```python
from build123d import *

# Parameters (mm, degrees)
BOSS_EXTRU_1_DEPTH           = 38
BOSS_EXTRU_1_DEPTH_BACK      = 10
ESQUISSE8_W                  = 200
ESQUISSE8_H                  = 45
ENL_V_MAT_EXTRU_4_DEPTH      = 34
TROU_TARAUD_M14X1_51_D       = 12.5
TROU_TARAUD_M14X1_51_DEPTH   = 17.5
TROU_TARAUD_M14X1_51_TIP     = 3.755378869
ESQUISSE10_W                 = 99
ESQUISSE10_H                 = 34
ENL_V_MAT_EXTRU_6_DEPTH      = 14
CONG_2_R                     = 10
ENL_V_MAT_EXTRU_7_DEPTH      = 1
ENL_V_MAT_EXTRU_7_DEPTH_BACK = 49
TROU_TARAUD_M12X1_251_D      = 10.8
CHANFREIN1_SIZE              = 3
CONG_3_R                     = 1
ESQUISSE14_W                 = 218.12810102
ESQUISSE14_H                 = 78.447864133
ENL_V_MAT_EXTRU_8_DEPTH      = 1


with BuildPart() as part:
    # Esquisse1 → Boss.-Extru.1 (new body, two sides)
    with BuildSketch(Plane(origin=(0, 0, 0), x_dir=(1, 0, 0), z_dir=(0, 1, 0))) as boss_extru_1_sk:
        with BuildLine():
            Line((-7.5, 31), (149.5, 31))
            Line((149.5, 31), (149.5, 17.146428199))
            ThreePointArc((149.5, 17.146428199), (150.241799002, 13.366783469), (152.357142857, 10.147886077))
            ThreePointArc((152.357142857, 10.147886077), (149.361144189, -12.492540023), (128.104434711, -4.142857143))
            ThreePointArc((128.104434711, -4.142857143), (124.497429283, 1.017837257), (118.521286236, 3))
            Line((118.521286236, 3), (23.478713764, 3))
            ThreePointArc((23.478713764, 3), (17.502570717, 1.017837257), (13.895565289, -4.142857143))
            ThreePointArc((13.895565289, -4.142857143), (-7.361144189, -12.492540023), (-10.357142857, 10.147886077))
            ThreePointArc((-10.357142857, 10.147886077), (-8.241799002, 13.366783469), (-7.5, 17.146428199))
            Line((-7.5, 17.146428199), (-7.5, 31))
        make_face()
    extrude(amount=BOSS_EXTRU_1_DEPTH)
    extrude(boss_extru_1_sk.sketch, amount=-BOSS_EXTRU_1_DEPTH_BACK)

    # Esquisse8 → Enlèv. mat.-Extru.4 (cut)
    with BuildSketch(Plane.XZ.offset(10)):
        with Locations((75, 4.5)):
            Rectangle(ESQUISSE8_W, ESQUISSE8_H)
    extrude(amount=-ENL_V_MAT_EXTRU_4_DEPTH, mode=Mode.SUBTRACT)

    # Trou taraudé M14x1.51
    with Locations(Plane(origin=(0, 0, -31), x_dir=(-1, 0, 0), z_dir=(0, 0, -1))):
        with Locations((-136, 19.5), (-6, 19.5)):
            Hole(TROU_TARAUD_M14X1_51_D / 2, depth=TROU_TARAUD_M14X1_51_DEPTH)
            with Locations((0, 0, -(TROU_TARAUD_M14X1_51_DEPTH + TROU_TARAUD_M14X1_51_TIP / 2))):  # 118° drill point
                Cone(0, TROU_TARAUD_M14X1_51_D / 2, TROU_TARAUD_M14X1_51_TIP, mode=Mode.SUBTRACT)

    # Esquisse10 → Enlèv. mat.-Extru.6 (cut, through all)
    with BuildSketch(Plane.XY.offset(-18)):
        with Locations((71, 7)):
            Rectangle(ESQUISSE10_W, ESQUISSE10_H)
    extrude(amount=-ENL_V_MAT_EXTRU_6_DEPTH, mode=Mode.SUBTRACT)

    # Congé2
    cong_2_edges = [part.edges().sort_by_distance(p)[0] for p in [
        (21.5, 24, -24.5),
        (120.5, 24, -24.5),
    ]]
    fillet(cong_2_edges, radius=CONG_2_R)

    # Esquisse11 → Enlèv. mat.-Extru.7 (cut, two sides)
    with BuildSketch(Plane(origin=(0, 38, 0), x_dir=(1, 0, 0), z_dir=(0, 1, 0))) as enl_v_mat_extru_7_sk:
        with BuildLine():
            Line((29.5, 27), (112.5, 27))
            ThreePointArc((112.5, 27), (119.571067812, 29.928932188), (122.5, 37))
            Line((122.5, 37), (122.5, 47))
            Line((122.5, 47), (19.5, 47))
            Line((19.5, 47), (19.5, 37))
            ThreePointArc((19.5, 37), (22.428932188, 29.928932188), (29.5, 27))
        make_face()
    extrude(amount=ENL_V_MAT_EXTRU_7_DEPTH, mode=Mode.SUBTRACT)
    extrude(enl_v_mat_extru_7_sk.sketch, amount=-ENL_V_MAT_EXTRU_7_DEPTH_BACK, mode=Mode.SUBTRACT)

    # Trou taraudé M12x1.251 (through all)
    with Locations(Plane(origin=(0, 24, 0), x_dir=(-1, 0, 0), z_dir=(0, -1, 0))):
        with Locations((0, 0), (-142, 0)):
            Hole(TROU_TARAUD_M12X1_251_D / 2)

    # Chanfrein1
    chanfrein1_edges = [part.edges().sort_by_distance(p)[0] for p in [
        (21.5, -10, -24.5),
        (120.5, -10, -24.5),
        (-7.5, -10, -24.5),
        (149.5, -10, -24.5),
    ]]
    chamfer(chanfrein1_edges, length=CHANFREIN1_SIZE)

    # Congé3
    cong_3_edges = [part.edges().sort_by_distance(p)[0] for p in [
        (144.918668947, 24, -18),
        (121.081331053, 24, -18),
        (20.918668947, 24, -18),
        (-2.918668947, 24, -18),
    ]]
    fillet(cong_3_edges, radius=CONG_3_R)

    # Esquisse14 → Enlèv. mat.-Extru.8 (cut)
    with BuildSketch(Plane(origin=(0, 38, 0), x_dir=(1, 0, 0), z_dir=(0, 1, 0))):
        with Locations((74.423535218, 6.641931997)):
            Rectangle(ESQUISSE14_W, ESQUISSE14_H)
    extrude(amount=-ENL_V_MAT_EXTRU_8_DEPTH, mode=Mode.SUBTRACT)


solid = part.part
```
Source: CAD feature listing. Evaluate the final solid. Frame: model axes, mm. A direction names the side the tool comes from. Give positions to 0.01 mm unless a question says otherwise; leave off trailing zeros. Loops run counter-clockwise (first coordinate to the right, second up) from the corner with the lowest first, then second, coordinate; pieces in that order, holes last. Notation, with made-up numbers: M 70,73 L 103,73 A18 cw 103,99 Z; hole C 49.5,35 d7. An arc over 180 degrees is marked long. Put each result on its own line as item: value.
Q1. Section D-D (x = 84). Return the cut outline in (y, z), and give its area (3 significant figures).
Response values:
outline: M 24,-27 L 37,-27 L 37,-3 L 24,-3 Z
area: 312 mm²
Q2. Pin query (flat end, axial travel): P1, Ø10.5, axis at x = 83, y = 30, coming from the -Z side; P2, Ø12, axis at x = 106.5, z = -20, coming from the -Y side; P3, Ø11, axis at x = 6, y = 19.5, coming from the -Z side. Return the tip coordinate at first contact, or that it passes through.
Response values:
P1: stops at z = -27
P2: stops at y = 23.8
P3: stops at z = -13.05
Q3. Reachability of faces 1 (the flat face through (136, 6, -18)), 2 (the cylindrical face through (124.569, 30.591, -0.964)), 3 (the cylindrical face through (117.65, 20.99, -24.1)), 4 (the cylindrical face through (139.36, 24.77, -24.07)) from +Z, -Z, +X, -X, +Y, -Y: full face, straight path, thin tool, end or side. Return the list, or none.
Response values:
face 1: +Z, +X, -X, -Y
face 2: +Z, +Y, -Y
face 3: +Z, -Z, -Y
face 4: -Z
Q4. Mould query, pull axis X, two halves, no side actions, for faces 5 (the cylindrical face through (116.914, 28.217, -28.027)), 6 (the flat face through (149.5, 15, -24)), 7 (the flat face through (10, 14, -31)), 8 (the flat face through (70, 30, -27)). Classes: released by +X, released by -X, zero draft, split by the parting line, or undercut.
Response values:
face 5: undercut
face 6: released by +X
face 7: zero draft
face 8: undercut
Q5. Section B-B (z = 8.5). Return the cut outline in (x, y).
Response values:
outline: M -11.75,24 L 11.75,24 L 11.75,37 L -11.75,37 Z; M 130.25,24 L 153.75,24 L 153.75,37 L 130.25,37 Z
Q6. Line query: probe 1 along Z at (x, y) = (0, 31.75); probe 2 along X at (y, z) = (25, -16); probe 3 along X at (y, z) = (8, -22). Output: solid intervals per line, ascending. Write a range as [from, to].
Response values:
probe 1: z = [-31, -5.4], [5.4, 14.5]
probe 2: x = [-7.57, 3.03], [8.97, 133.03], [138.97, 149.57]
probe 3: x = [-7.5, 21.5], [120.5, 149.5]
Q7. Section A-A (y = 28.5). Return the cut outline in (x, z).
Response values:
outline: M -10.36,-10.15 A10 cw -7.5,-17.15 L -7.5,-31 L 21.5,-31 A10 cw 29.5,-27 L 112.5,-27 A10 cw 120.5,-31 L 149.5,-31 L 149.5,-17.15 A10 cw 152.36,-10.15 A14.5 ccw long 128.1,4.14 A10 cw 118.52,-3 L 23.48,-3 A10 cw 13.9,4.14 A14.5 ccw long Z; hole C 0,0 d10.8; hole C 142,0 d10.8
Q8. Section C-C (z = 2). Return the cut outline in (x, y), and give its area (3 significant figures).
Response values:
outline: M -14.36,24 L -5.02,24 L -5.02,37 L -14.36,37 Z; M 5.02,24 L 14.82,24 L 14.82,37 L 5.02,37 Z; M 127.18,24 L 136.98,24 L 136.98,37 L 127.18,37 Z; M 147.02,24 L 156.36,24 L 156.36,37 L 147.02,37 Z
area: 498 mm²
